Autodesk Inventor part; units mm, degrees
ref_plane "YZ Plane" through (0, 0, 0) normal (1, 0, 0) x (0, 1, 0)
ref_plane "XZ Plane" through (0, 0, 0) normal (0, 1, 0) x (-1, 0, 0)
ref_plane "XY Plane" through (0, 0, 0) normal (0, 0, 1) x (1, 0, 0)
sketch "Sketch1" plane through (0, 0, 0) normal (0, 0, 1) x (1, 0, 0)
  circle A0 centre (0, -25) radius 1.25 construction
  circle A1 centre (0, 25) radius 1.25 construction
  circle A2 centre (0, 0) radius 1.25 construction
  line L0 (6, 28.3) -> (11, 33.3) construction
  line L1 (11, 33.3) -> (11, 41.3) construction
  line L2 (9, 43.3) -> (-9, 43.3) construction
  line L3 (-11, 41.3) -> (-11, 33.3) construction
  line L4 (-11, 33.3) -> (-6, 28.3) construction
  line L5 (-6, 28.3) -> (-6, -28.3) construction
  line L6 (-6, -28.3) -> (-11, -33.3) construction
  line L7 (-11, -33.3) -> (-11, -41.3) construction
  line L8 (-9, -43.3) -> (9, -43.3) construction
  line L9 (11, -41.3) -> (11, -33.3) construction
  line L10 (11, -33.3) -> (6, -28.3) construction
  line L11 (6, -28.3) -> (6, 28.3) construction
  circle A3 centre (-6, -38.3) radius 1.375 construction
  circle A4 centre (6, -38.3) radius 1.375 construction
  circle A5 centre (6, 38.3) radius 1.375 construction
  circle A6 centre (-6, 38.3) radius 1.375 construction
  line L12 (13.5, 47.5) -> (13.5, -47.5) construction
  line L13 (-8, -31) -> (13.5, -31)
  line L14 (13.5, -31) -> (13.5, 31)
  line L15 (13.5, 31) -> (-8, 31)
  line L16 (-8, 31) -> (-8, -31)
  arc A7 (11, 41.3) -> (9, 43.3) centre (9, 41.3) ccw
  arc A8 (-9, 43.3) -> (-11, 41.3) centre (-9, 41.3) ccw
  arc A9 (-11, -41.3) -> (-9, -43.3) centre (-9, -41.3) ccw
  arc A10 (9, -43.3) -> (11, -41.3) centre (9, -41.3) ccw
  point P0 (0, 0)
  dimension "d0" = 6
  dimension "d1" = 6
  dimension "d2" = 8
extrude "Extrusion1" add sketch "Sketch1" along normal blind 10
shell "Shell1" thickness 2 removed faces 4 at (-0.8333, -31, 3.3333) at (-8, 10.3333, 3.3333) at (-0.8333, 10.3333, 10) at (6.3333, 31, 3.3333)
sketch "Sketch2" plane through (11.5, -31, 2) normal (-1, 0, 0) x (0, 0, 1)
  circle A0 centre (3.075, 10.3598) radius 1.25 construction
  circle A1 centre (3.075, 51.6402) radius 1.25 construction
  line L0 (0, 0) -> (0, 62)
  line L1 (8, 0) -> (0, 0)
  line L2 (8, 62) -> (8, 0)
  line L3 (0, 62) -> (8, 62)
  line L4 (1.575, 10.3598) -> (4.575, 10.3598) construction
  line L5 (1.575, 9.2348) -> (4.575, 9.2348)
  line L6 (4.575, 11.4848) -> (1.575, 11.4848)
  arc A2 (1.575, 11.4848) -> (1.575, 9.2348) centre (1.575, 10.3598) ccw
  arc A3 (4.575, 9.2348) -> (4.575, 11.4848) centre (4.575, 10.3598) ccw
  line L7 (1.575, 51.6402) -> (4.575, 51.6402) construction
  line L8 (1.575, 50.5152) -> (4.575, 50.5152)
  line L9 (4.575, 52.7652) -> (1.575, 52.7652)
  arc A4 (1.575, 52.7652) -> (1.575, 50.5152) centre (1.575, 51.6402) ccw
  arc A5 (4.575, 50.5152) -> (4.575, 52.7652) centre (4.575, 51.6402) ccw
  line L10 (3.075, 51.6402) -> (6.075, 51.6402) construction
  point P0 (-2, 31)
  dimension "d6" = 1.5
  dimension "d7" = 2.25
  dimension "d8" = 1.5
  dimension "d9" = 0
  dimension "d10" = 2.25
extrude "Extrusion2" cut sketch "Sketch2" against normal through all contours A2 L6 A3 L5 | A4 L9 A5 L8
sketch "Sketch3" plane through (-8, 31, 2) normal (0, 0, 1) x (1, 0, 0)
  circle A0 centre (8, -56) radius 1.25
  circle A1 centre (8, -6) radius 1.25
  circle A2 centre (8, -31) radius 1.25
  line L0 (14, -2.7) -> (19, 2.3)
  line L1 (19, 2.3) -> (19, 10.3)
  line L2 (17, 12.3) -> (-1, 12.3)
  line L3 (-3, 10.3) -> (-3, 2.3)
  line L4 (-3, 2.3) -> (2, -2.7)
  line L5 (2, -2.7) -> (2, -59.3)
  line L6 (2, -59.3) -> (-3, -64.3)
  line L7 (-3, -64.3) -> (-3, -72.3)
  line L8 (-1, -74.3) -> (17, -74.3)
  line L9 (19, -72.3) -> (19, -64.3)
  line L10 (19, -64.3) -> (14, -59.3)
  line L11 (14, -59.3) -> (14, -2.7)
  circle A3 centre (2, -69.3) radius 1.375
  circle A4 centre (14, -69.3) radius 1.375
  circle A5 centre (14, 7.3) radius 1.375
  circle A6 centre (2, 7.3) radius 1.375
  arc A7 (19, 10.3) -> (17, 12.3) centre (17, 10.3) ccw
  arc A8 (-1, 12.3) -> (-3, 10.3) centre (-1, 10.3) ccw
  arc A9 (-3, -72.3) -> (-1, -74.3) centre (-1, -72.3) ccw
  arc A10 (17, -74.3) -> (19, -72.3) centre (17, -72.3) ccw
  point P0 (8, -31)
extrude "Extrusion3" cut sketch "Sketch3" against normal through all contours A0 | A1 | A2
sketch "Sketch4" plane through (-8, 31, 2) normal (0, 0, 1) x (1, 0, 0)
  line L0 (19.5, -52.7652) -> (19.5, -50.5152)
  line L1 (19.5, -11.4848) -> (19.5, -9.2348)
  line L2 (19.5, -62) -> (19.5, 0) construction
  line L3 (19.5, -57.1304) -> (15.5, -55.2652)
  line L4 (15.5, -55.2652) -> (15.5, -48.0152)
  line L5 (15.5, -48.0152) -> (19.5, -46.1499)
  line L6 (19.5, -52.7652) -> (15.5, -52.7652) construction
  line L7 (19.5, -50.5152) -> (15.5, -50.5152) construction
  line L8 (19.5, -57.1304) -> (19.5, -46.1499)
  point P0 (8, -31)
  dimension "d15" = 65
  dimension "d16" = 65
  dimension "d18" = 2.5
  dimension "d19" = 2.5
  dimension "d20" = 4
extrude "Extrusion4" cut sketch "Sketch4" against normal through all
sketch "Sketch5" plane through (-8, 31, 2) normal (0, 0, 1) x (1, 0, 0)
  line L0 (15.5, -48.0152) -> (19.5, -46.1499)
  line L1 (19.5, -46.1499) -> (19.5, 0)
  line L2 (0, 0) -> (19.5, 0)
  line L3 (0, -62) -> (0, 0)
  line L4 (19.5, -62) -> (0, -62)
  line L5 (19.5, -62) -> (19.5, -57.1304)
  line L6 (19.5, -57.1304) -> (15.5, -55.2652)
  line L7 (15.5, -55.2652) -> (15.5, -48.0152)
  circle A0 centre (8, -6) radius 1.25
  circle A1 centre (8, -31) radius 1.25
  circle A2 centre (8, -56) radius 1.25
  line L8 (0, -52) -> (4, -50.1348)
  line L9 (4, -50.1348) -> (4, -11.8652)
  line L10 (4, -11.8652) -> (0, -10)
  point P0 (8, -31)
  dimension "d25" = 10
  dimension "d26" = 65
  dimension "d27" = 65
  dimension "d28" = 10
  dimension "d29" = 4
extrude "Extrusion5" cut sketch "Sketch5" against normal through all contours L10 L9 L8 L3
mirror "Mirror1" about plane through (0, 0, 0) normal (0, 1, 0) of "Extrusion4"
sketch "Sketch7" plane through (11.5, -31, 10) normal (-1, 0, 0) x (0, 0, 1)
  line L0 (-6.425, 52.7652) -> (-3.425, 52.7652)
  arc A0 (-3.425, 50.5152) -> (-3.425, 52.7652) centre (-3.425, 51.6402) ccw
  line L1 (-3.425, 50.5152) -> (-6.425, 50.5152)
  arc A1 (-6.425, 52.7652) -> (-6.425, 50.5152) centre (-6.425, 51.6402) ccw
  line L2 (-6.425, 11.4848) -> (-3.425, 11.4848)
  arc A2 (-3.425, 9.2348) -> (-3.425, 11.4848) centre (-3.425, 10.3598) ccw
  line L3 (-3.425, 9.2348) -> (-6.425, 9.2348)
  arc A3 (-6.425, 11.4848) -> (-6.425, 9.2348) centre (-6.425, 10.3598) ccw
  line L4 (-8, 0) -> (-8, 4.8696)
  line L5 (0, 0) -> (-8, 0)
  line L6 (0, 62) -> (0, 0)
  line L7 (-8, 62) -> (0, 62)
  line L8 (-8, 57.1304) -> (-8, 62)
  line L9 (-8, 57.1304) -> (-10, 57.1304)
  line L10 (-10, 46.1499) -> (-10, 57.1304)
  line L11 (-8, 46.1499) -> (-10, 46.1499)
  line L12 (-8, 15.8501) -> (-8, 46.1499)
  line L13 (-8, 15.8501) -> (-10, 15.8501)
  line L14 (-10, 4.8696) -> (-10, 15.8501)
  line L15 (-8, 4.8696) -> (-10, 4.8696)
  line L16 (0, 0) -> (0, 62)
  line L17 (0, 31) -> (-8, 31)
  line L18 (0, 32) -> (-8, 32)
  line L19 (0, 30) -> (-8, 30)
  point P0 (-10, 31)
  dimension "d32" = 1
  dimension "d33" = 1
extrude "Extrusion6" add sketch "Sketch7" along normal blind 6 contours L19 L12 L17 L6 | L17 L12 L18 L6
draft "FaceDraft1" angle 25 pull direction (0, 0, 1) faces at (5.5, 0.3333, 4.6667) fixed edges at (5.5, 0, 2)
pattern_linear "Rectangular Pattern1" count 5 spacing 6 along (0, -1, 0) of "Extrusion6", "FaceDraft1" first direction both ways yes
fillet "Fillet1" radius 2 4 edges at (-8, -31, 1) (-8, 31, 1) (12.5, 31, 10) (12.5, -31, 10)
equation "\"d1\" = d0"
equation "\"d7\" = d10"
equation "\"d16\" = d15"
equation "\"d19\" = d18"
equation "\"d27\" = d26"
equation "\"d28\" = d25"
equation "\"d33\" = d32"
properties part number "A-07"
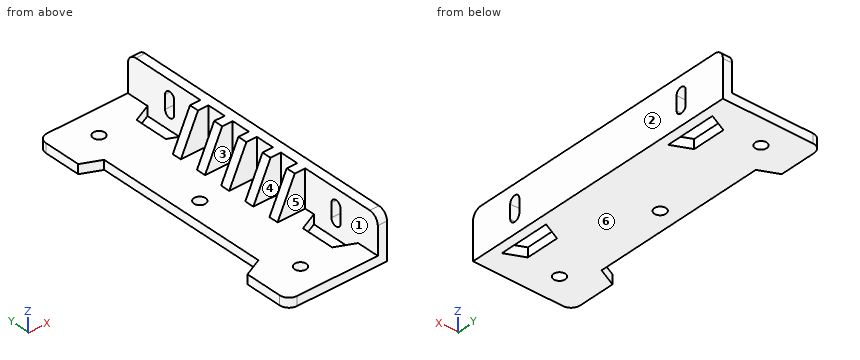
Check sheet for the modelled part. Datum: model origin and axes. Units: mm. Face numbers are marked on the shaded views. A direction names the side the tool comes from. Coordinates: 2 decimals unless noted, no trailing zeros. Loops run counter-clockwise (first coordinate to the right, second up) from the corner with the lowest first, then second, coordinate; pieces in that order, holes last.
1) Gauge pin test, flat ends, axial feed: pin 1 (2 mm diameter, centred on x = 6, z = 7.5, fed in from +Y); pin 2 (3 mm diameter, centred on x = 9, z = 5.5, fed in from -Y); pin 3 (1.2 mm diameter, centred on y = 8, z = 8, fed in from -X); pin 4 (1.8 mm diameter, centred on x = 7.5, z = 8, fed in from +Y). Record the tip position at first contact, or that the pin passes through.
2) Release check for a two-part mould opening along Y. For the marked faces 4, 5 and 6 record: released by +Y, released by -Y, zero draft, split by the parting line, or undercut.
3) Sectioned sample at C-C (x = 0). Record the boundary of the cut face in (y, z), and give its area (3 significant figures).
4) Material ranges on probe 1 along Y at (x, z) = (0, 1.25); probe 2 along Z at (x, y) = (0.75, -21.5); probe 3 along X at (y, z) = (-22, 6), recorded low to high.
5) Access from +Z, -Z, +X, -X, +Y, -Y to the whole of each face (thin tool, end or side, straight path). Record for the marked faces 1, 2 and 3.
6) Sectioned sample at D-D (z = 6). Count the separate pieces of the cut face and the enclosed holes in it, and give its area (3 significant figures).
7) Sectioned sample at A-A (y = 0). Record the boundary of the cut face in (x, z).
8) Sectioned sample at B-B (z = 1). Record the boundary of the cut face in (x, y).
Check sheet entries:
1. pin 1: passes through
1. pin 2: stops at y = -13
1. pin 3: stops at x = 11.5
1. pin 4: stops at y = 13
2. face 4: undercut
2. face 5: released by -Y
2. face 6: zero draft
3. outline: (-31, 0) - (-26.25, 0) - (-26.25, 2) - (-31, 2) - close; (-23.75, 0) - (-1.25, 0) - (-1.25, 2) - (-23.75, 2) - close; (1.25, 0) - (23.75, 0) - (23.75, 2) - (1.25, 2) - close; (26.25, 0) - (31, 0) - (31, 2) - (26.25, 2) - close
3. area: 109 mm2
4. probe 1: y = -31 to -26.25, -23.75 to -1.25, 1.25 to 23.75, 26.25 to 31
4. probe 2: z = 0 to 2
4. probe 3: x = 11.5 to 13.5
5. face 1: +Z
5. face 2: +Z, -Z, +X, +Y, -Y
5. face 3: +Z, -X
6. separate pieces: 3
6. enclosed holes: 0
6. area: 156 mm2
7. outline: (-4, 0) - (-1.25, 0) - (-1.25, 2) - (-4, 2) - close; (1.25, 0) - (13.5, 0) - (13.5, 10) - (9.23, 10) - (5.5, 2) - (1.25, 2) - close
8. outline: (-8, -29) arc R2 ccw to (-6, -31) - (13.5, -31) - (13.5, 31) - (-6, 31) arc R2 ccw to (-8, 29) - (-8, 21) - (-4, 19.13) - (-4, -19.13) - (-8, -21) - close; hole circle Ø2.5 at (0, -25); hole circle Ø2.5 at (0, 0); hole circle Ø2.5 at (0, 25); hole (7.5, -24.27) - (11.5, -26.13) - (11.5, -15.15) - (7.5, -17.02) - close; hole (7.5, 17.02) - (11.5, 15.15) - (11.5, 26.13) - (7.5, 24.27) - close
